Source: CAD feature listing. Evaluate the final solid. Frame: model axes, mm. A direction names the side the tool comes from. Coordinates: 2 decimals unless noted, no trailing zeros. Order: outer loops, then holes, each group sorted by start corner. A loop starts at its lowest first (then second) coordinate and runs counter-clockwise, first axis right, second up.
Item 1: Ray query, line 1 (X direction, y = 15, z = 21.5) (3 decimals); line 2 (Y direction, x = 7, z = 15) (3 decimals); line 3 (Z direction, x = 65.5, y = 3) (3 decimals). Return the intervals inside material, ascending.
Item 2: Reachability of faces 1 (the flat face through (-5, -3.175, 31)), 2 (the flat face through (98, 19.05, 53)), 3 (the flat face through (54, 25.4, 45)) from +Z, -Z, +X, -X, +Y, -Y: full face, straight path, thin tool, end or side. Return the list, or none.
Item 3: Mould query, pull axis X, two halves, no side actions, for faces 4 (the cylindrical face through (32.73, -14.44, 51.97)), 5 (the cylindrical face through (45.8, -0.4, 38.1)), 6 (the cylindrical face through (0.58, -61.97, -8.08)). Classes: released by +X, released by -X, zero draft, split by the parting line, or undercut.
Item 4: Section D-D on x = 80.5. Return the cut outline in (y, z) (3 decimals).
Item 5: Section C-C on y = -32. Return the cut outline in (x, z) (3 decimals), then the cut area to 3 significant figures.
Item 6: Contact query for flat-ended pins moving along their axis: P1, Ø2, axis at x = 63, y = 27, coming from the -Z side; P2, Ø7, axis at y = -23, z = 1, coming from the -X side (3 decimals); P3, Ø14, axis at y = 13, z = 22.5, coming from the -X side (3 decimals); P4, Ø1, axis at x = 58, y = -10.5, coming from the -Z side. Output: stop coordinate, or through.
Item 7: Section A-A on y = 9. Return the cut outline in (x, z) (3 decimals), then the cut area to 3 significant figures.
Item 8: Section B-B on x = 96. Return the cut outline in (y, z) (3 decimals).
from build123d import *

# Parameters (mm, degrees)
F1_DEPTH = 63.5
F0_W     = 25.4
F0_H     = 19.05
F0_H_2   = 4.7498
F0_H_3   = 4.7752
F2_DEPTH = 25.4
F3_DEPTH = 3.175
F4_R     = 5.08
F5_DEPTH = 19.05


with BuildPart() as f1:
    # F0 (on Front) → F1 (new body, symmetric)
    with BuildSketch(Plane.XZ):
        Polygon((-41.275, -9.525), (41.275, -9.525), (41.275, 9.525), (22.225, 9.525), (-41.275, 9.525), align=None)
    extrude(amount=F1_DEPTH, both=True)

    # F0 (on Front) → F2 (join, symmetric)
    with BuildSketch(Plane.XZ):
        with BuildLine():
            Line((22.225, 9.525), (41.275, 9.525))
            Line((41.275, 9.525), (41.275, 27.0002))
            ThreePointArc((41.275, 27.0002), (45.9246798487, 38.2255201513), (57.15, 42.8752))
            Line((57.15, 42.8752), (60.325, 42.8752))
            Line((60.325, 42.8752), (60.325, 61.9252))
            Line((60.325, 61.9252), (57.15, 61.9252))
            ThreePointArc((57.15, 61.9252), (32.4542956671, 51.6959043329), (22.225, 27.0002))
            Line((22.225, 27.0002), (22.225, 9.525))
        make_face()
        with Locations((73.025, 52.4002)):
            Rectangle(F0_W, F0_H)
        with Locations((73.025, 64.3001)):
            Rectangle(F0_W, F0_H_2)
        with Locations((73.025, 40.4876)):
            Rectangle(F0_W, F0_H_3)
    extrude(amount=F2_DEPTH, both=True)

    # F0 (on Front) → F3 (join, symmetric)
    with BuildSketch(Plane.XZ):
        with BuildLine():
            add(Edge.make_bspline(
                [(-41.275, 9.525), (-46.2452806532, 64.7963359952), (25.8592385799, 62.7934262156), (57.15, 61.9252)],
                knots=[0, 0, 0, 0, 111.5045361635, 111.5045361635, 111.5045361635, 111.5045361635], degree=3))
            Line((-41.275, 9.525), (22.225, 9.525))
            Line((22.225, 9.525), (22.225, 27.0002))
            ThreePointArc((22.225, 27.0002), (32.4542956671, 51.6959043329), (57.15, 61.9252))
        make_face()
    extrude(amount=F3_DEPTH, both=True)

    # F4
    f4_edges = [f1.edges().sort_by_distance(p)[0] for p in [
        (0, -63.5, -9.525),
        (41.275, 0, -9.525),
        (0, 63.5, -9.525),
        (-41.275, 0, -9.525),
    ]]
    fillet(f4_edges, radius=F4_R)

    # F0 (on Front) → F5 (join, symmetric)
    with BuildSketch(Plane.XZ):
        Polygon((85.725, 66.675), (85.725, 61.9252), (85.725, 42.8752), (85.725, 38.1), (111.125, 38.1), (111.125, 66.675), align=None)
    extrude(amount=F5_DEPTH, both=True)


solid = f1.part
Answer list:
1. line 1: x = 22.225 to 41.275
1. line 2: y = -3.175 to 3.175
1. line 3: z = 38.1 to 66.675
2. face 1: +Z, -X, -Y
2. face 2: +Z, -Z, +X, +Y
2. face 3: +Z, +X, -X, +Y
3. face 4: released by -X
3. face 5: undercut
3. face 6: zero draft
4. outline: (-25.4, 38.1) - (25.4, 38.1) - (25.4, 66.675) - (-25.4, 66.675) - close
5. outline: (-41.275, -4.445) arc R5.08 ccw to (-36.195, -9.525) - (36.195, -9.525) arc R5.08 ccw to (41.275, -4.445) - (41.275, 9.525) - (-41.275, 9.525) - close
5. area: 1,560 mm2
6. P1: passes through
6. P2: stops at x = -41.275
6. P3: stops at x = 22.225
6. P4: stops at z = 42.88
7. outline: (-41.275, -4.445) arc R5.08 ccw to (-36.195, -9.525) - (36.195, -9.525) arc R5.08 ccw to (41.275, -4.445) - (41.275, 27) arc R15.875 cw to (57.15, 42.875) - (60.325, 42.875) - (60.325, 38.1) - (111.125, 38.1) - (111.125, 66.675) - (60.325, 66.675) - (60.325, 61.925) - (57.15, 61.925) arc R34.925 ccw to (22.225, 27) - (22.225, 9.525) - (-41.275, 9.525) - close
7. area: 4,170 mm2
8. outline: (-19.05, 38.1) - (19.05, 38.1) - (19.05, 66.675) - (-19.05, 66.675) - close
